Source: CAD feature listing. Evaluate the final solid. Frame: model axes, mm. A direction names the side the tool comes from. Round coordinates to 2 decimals unless told otherwise and drop trailing zeros.
Item 1: Access query for faces 1 (the flat face through (30, 108.091, -111)), 2 (the cylindrical face through (50.14, 102.22, -205.85)). Directions: +Z, -Z, +X, -X, +Y, -Y. A direction counts if a zero-diameter tool reaches every point of the face in a straight line with its end or side. Return the directions, or none.
Item 2: Ray query, L1, parallel to Z at x = 53.5, y = 101.5; L2, parallel to Y at x = 40.5, z = -201.5. Return the intervals inside material, ascending.
Item 3: Pull-direction query (Y, two-part tool) for faces 3 (the flat face through (40, 101, -202)), 4 (the flat face through (30, -1.909, -111)), 5 (the flat face through (60, 54, -111)); classes: released by +Y, released by -Y, zero draft, split by the parting line, or undercut.
Item 4: First-contact query: P1, Ø7, axis at y = 101.02, z = -202.03, coming from the +X side. Flat tip, straight axial feed; report the tip coordinate or a pass-through.
```python
from build123d import *

# Parameters (mm, degrees)
SKETCH_1_W          = 200
SKETCH_1_H          = 110
EXTRUDE_1_DEPTH     = 60
SKETCH_3_R          = 4
CUT_EXTRUDE_2_DEPTH = 20


with BuildPart() as part:
    # Эскиз1 → Бобышка-Вытянуть1 (new body)
    with BuildSketch(Plane(origin=(0, 0, 0), x_dir=(0, 0, -1), z_dir=(1, 0, 0))):
        with Locations((111.99379123, 53.09072323)):
            Rectangle(SKETCH_1_W, SKETCH_1_H)
    extrude(amount=EXTRUDE_1_DEPTH)

    # Эскиз3 → Вырез-Вытянуть2 (cut)
    with BuildSketch(Plane(origin=(60, 0, 0), x_dir=(0, 0, -1), z_dir=(1, 0, 0))):
        with Locations((202.033930041, 101.016084536)):
            Circle(SKETCH_3_R)
    extrude(amount=-CUT_EXTRUDE_2_DEPTH, mode=Mode.SUBTRACT)


solid = part.part
```
Data:
1. face 1: +Z, -Z, +X, -X, +Y
1. face 2: +X
2. L1: z = -211.99 to -206, -198.06 to -11.99
2. L2: y = -1.91 to 97.05, 104.98 to 108.09
3. face 3: undercut
3. face 4: released by -Y
3. face 5: zero draft
4. P1: stops at x = 40
